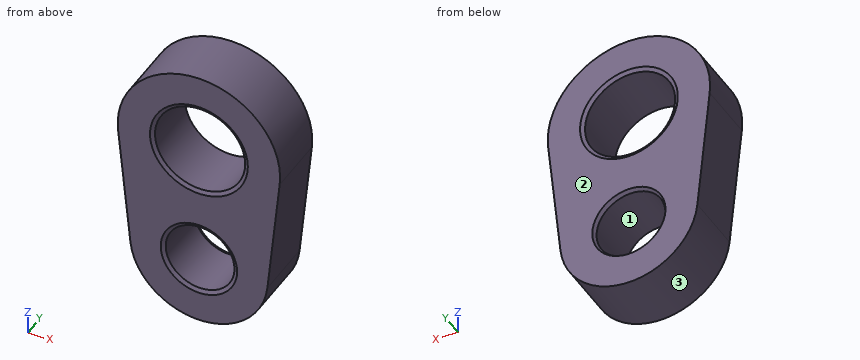
from build123d import *

# Parameters (mm, degrees)
F0_R        = 1.9812
F0_R_2      = 2.59715
F1_DEPTH    = 3.4544
F2_C1_SIZE2 = 0.127
F2_C1_SIZE  = 0.2199704526
F2_C2_SIZE2 = 0.2199704526
F2_C2_SIZE  = 0.127
F2_C3_SIZE2 = 0.127
F2_C3_SIZE  = 0.2199704526
F2_C4_SIZE2 = 0.2199704526
F2_C4_SIZE  = 0.127


with BuildPart() as f1:
    # F0 (on Front) → F1 (new body)
    with BuildSketch(Plane.XZ):
        with BuildLine():
            Line((-4.6498341341, -0.4707223022), (-3.9422506789, -7.4602906475))
            ThreePointArc((-3.9422506789, -7.4602906475), (0, -11.0236), (3.9422506789, -7.4602906475))
            Line((3.9422506789, -7.4602906475), (4.6498341341, -0.4707223022))
            ThreePointArc((4.6498341341, -0.4707223022), (0, 4.6736), (-4.6498341341, -0.4707223022))
        make_face()
        with Locations((0, -7.0612)):
            Circle(F0_R, mode=Mode.SUBTRACT)
        Circle(F0_R_2, mode=Mode.SUBTRACT)
    extrude(amount=F1_DEPTH)

    # F2: chamfer of 0.127 x 0.2199704526 on 4 edges, made by hand

    # F2_c1
    f2_c1_edges = [f1.edges().sort_by_distance(p)[0] for p in [
        (-1.9812, 0, -7.0612),
    ]]
    f2_c1_side = f1.faces().sort_by_distance((-1.9812, -0.00254, -7.0612))[0]
    chamfer(f2_c1_edges, length=F2_C1_SIZE, length2=F2_C1_SIZE2, reference=f2_c1_side)

    # F2_c2
    f2_c2_edges = [f1.edges().sort_by_distance(p)[0] for p in [
        (-1.9812, -3.4544, -7.0612),
    ]]
    f2_c2_side = f1.faces().sort_by_distance((-1.9812, -3.45186, -7.0612))[0]
    chamfer(f2_c2_edges, length=F2_C2_SIZE, length2=F2_C2_SIZE2, reference=f2_c2_side)

    # F2_c3
    f2_c3_edges = [f1.edges().sort_by_distance(p)[0] for p in [
        (-2.59715, 0, 0),
    ]]
    f2_c3_side = f1.faces().sort_by_distance((-2.59969, 0, 0))[0]
    chamfer(f2_c3_edges, length=F2_C3_SIZE, length2=F2_C3_SIZE2, reference=f2_c3_side)

    # F2_c4
    f2_c4_edges = [f1.edges().sort_by_distance(p)[0] for p in [
        (-2.59715, -3.4544, 0),
    ]]
    f2_c4_side = f1.faces().sort_by_distance((-2.59715, -3.45186, 0))[0]
    chamfer(f2_c4_edges, length=F2_C4_SIZE, length2=F2_C4_SIZE2, reference=f2_c4_side)


solid = f1.part
The listing builds one solid part. Answer for the finished solid, in the listing's coordinates (mm). Face numbers are marked on the shaded views. Coordinates: 2 decimals unless noted, no trailing zeros. Write each loop counter-clockwise with the first axis right and the second up, starting at its lowest first coordinate (ties: lowest second). Pieces come first, ordered by that corner, then holes. Notation, with made-up numbers: (-2, 23) - (35, 23) arc R6 ccw to (35, 34) - close; hole circle Ø8 at (-19.5, 36). An arc over 180 degrees is marked (long way). Return JSON: item names as keys, results as strings.
1. The part is cut by section B-B on x = 0. Determine the outline of the cut face in (y, z), then the cut area to 3 significant figures.
Final values:
{"outline": "(-3.45, -11.02) - (0, -11.02) - (0, -9.17) - (-0.22, -9.04) - (-3.33, -9.04) - (-3.45, -9.26) - close; (-3.45, -4.86) - (-3.33, -5.08) - (-0.22, -5.08) - (0, -4.95) - (0, -2.82) - (-0.13, -2.6) - (-3.33, -2.6) - (-3.45, -2.82) - close; (-3.45, 2.82) - (-3.33, 2.6) - (-0.13, 2.6) - (0, 2.82) - (0, 4.67) - (-3.45, 4.67) - close", "area": "22.5 mm^2"}
2. For a pull along Z with two mould halves and no side action, classify the marked faces 1, 2 and 3 as +Z half, -Z half, draft (parallel to the pull), parting line (faces both ways), or undercut.
Final values:
{"face 1": "undercut", "face 2": "draft", "face 3": "-Z half"}
3. The part is cut by section D-D on x = -3.75. Determine the outline of the cut face in (y, z).
Final values:
{"outline": "(-3.45, -8.34) - (0, -8.34) - (0, 2.79) - (-3.45, 2.79) - close"}
4. Consider line 1 along Z through (x, y) = (0, -0.9); line 2 along Z through (x, y) = (-1.25, -3.2); line 3 along X through (y, z) = (-2.5, -2.25). Determine where each line is inside the solid, lowest interval first.
Final values:
{"line 1": "-11.02 to -9.04, -5.08 to -2.6, 2.6 to 4.67", "line 2": "-10.82 to -8.6, -5.52 to -2.28, 2.28 to 4.5", "line 3": "-4.47 to -1.3, 1.3 to 4.47"}
5. Each of these flat-tipped pins is pushed along its axis until it touches: pin 1 Ø4 at (x, z) = (2.5, 1.5) entering from +Y; pin 2 Ø4.5 at (x, z) = (0, 0) entering from -Y; pin 3 Ø1.5 at (x, y) = (-3.5, -1.5) entering from +Z. Where does it stop, or does it pass through?
Final values:
{"pin 1": "y = 0", "pin 2": "through", "pin 3": "z = 3.78"}
6. The part is cut by section C-C on y = -2.2. Determine the outline of the cut face in (x, z), then the cut area to 3 significant figures.
Final values:
{"outline": "(-4.65, -0.47) - (-3.94, -7.46) arc R3.96 ccw to (3.94, -7.46) - (4.65, -0.47) arc R4.67 ccw (long way) to start; hole circle Ø5.19 at (0, 0); hole circle Ø3.96 at (0, -7.06)", "area": "86.7 mm^2"}
7. The part is cut by section A-A on z = 0. Determine the outline of the cut face in (x, y), then the cut area to 3 significant figures.
Final values:
{"outline": "(-4.67, -3.45) - (-2.82, -3.45) - (-2.6, -3.33) - (-2.6, -0.13) - (-2.82, 0) - (-4.67, 0) - close; (2.6, -3.33) - (2.82, -3.45) - (4.67, -3.45) - (4.67, 0) - (2.82, 0) - (2.6, -0.13) - close", "area": "14.3 mm^2"}
